from build123d import *

# Parameters (mm, degrees)
F1_DEPTH = 25.4


with BuildPart() as f1:
    # F0 (on Front) → F1 (new body)
    with BuildSketch(Plane.XZ):
        with BuildLine():
            Line((-180.280449281, -69.793186067), (-37.9985533655, -73.516196597))
            Line((-37.9985533655, -73.516196597), (-37.9985533655, -53.3922091126))
            ThreePointArc((-37.9985533655, -53.3922091126), (-36.3574166334, -49.6531424612), (-32.4943724898, -48.3299496779))
            Line((-32.4943724898, -48.3299496779), (32.4792108915, -48.1490081299))
            ThreePointArc((32.4792108915, -48.1490081299), (36.3518127667, -49.4657614096), (37.9985533655, -53.209974262))
            Line((37.9985533655, -53.209974262), (37.9985533655, -73.516196597))
            Line((37.9985533655, -73.516196597), (180.280449281, -69.793186067))
            Line((180.280449281, -69.793186067), (179.7684819711, -50.3384282921))
            ThreePointArc((179.7684819711, -50.3384282921), (181.2076799987, -46.6602509384), (184.8467238815, -45.124790347))
            Line((184.8467238815, -45.124790347), (224.0474202454, -45.124790347))
            ThreePointArc((224.0474202454, -45.124790347), (227.6395226938, -46.6126878986), (229.1274202454, -50.204790347))
            Line((229.1274202454, -50.204790347), (229.1274202454, -68.8998913716))
            Line((229.1274202454, -68.8998913716), (368.779072779, -65.2248478839))
            Line((368.779072779, -65.2248478839), (368.2445209989, -44.9118802426))
            ThreePointArc((368.2445209989, -44.9118802426), (369.6374073208, -41.2818793035), (373.1891249642, -39.7000003873))
            Line((373.1891249642, -39.7000003873), (413.8150602467, -38.6308968272))
            ThreePointArc((413.8150602467, -38.6308968272), (417.4450611859, -40.0237831491), (419.0269401021, -43.5755007925))
            Line((419.0269401021, -43.5755007925), (419.5614918821, -63.8884684338))
            Line((419.5614918821, -63.8884684338), (572.7053844218, -59.8583659985))
            Line((572.7053844218, -59.8583659985), (571.7030998342, -21.7715516712))
            ThreePointArc((571.7030998342, -21.7715516712), (573.0959861561, -18.141550732), (576.6477037995, -16.5596718159))
            Line((576.6477037995, -16.5596718159), (593.6560001815, -16.112085069))
            add(Edge.make_bspline(
                [(593.6560001815, -16.112085069), (596.1080901801, 20.5341002257), (601.6949471336, 104.0289944805), (592.471101525, 224.502637459), (587.295632267, 292.1)],
                knots=[0, 0, 0, 0, 0.4389033081, 1, 1, 1, 1], degree=3))
            Line((587.295632267, 292.1), (561.895632267, 292.1))
            ThreePointArc((561.895632267, 292.1), (555.545632267, 298.45), (561.895632267, 304.8))
            Line((561.895632267, 304.8), (561.895632267, 317.5))
            Line((561.895632267, 317.5), (479.345632267, 330.2))
            Line((479.345632267, 330.2), (479.345632267, 266.595095396))
            add(Edge.make_bspline(
                [(479.345632267, 266.595095396), (537.2284650803, 211.8650227785), (542.5910949707, 164.6739989519), (523.795632267, 101.6)],
                knots=[0, 0, 0, 0, 170.8776872642, 170.8776872642, 170.8776872642, 170.8776872642], degree=3))
            Line((523.795632267, 101.6), (479.345632267, 0))
            Line((479.345632267, 0), (0, 0))
            Line((0, 0), (-479.345632267, 0))
            Line((-479.345632267, 0), (-523.795632267, 101.6))
            add(Edge.make_bspline(
                [(-479.345632267, 266.595095396), (-537.2284650803, 211.8650227785), (-542.5910949707, 164.6739989519), (-523.795632267, 101.6)],
                knots=[0, 0, 0, 0, 170.8776872642, 170.8776872642, 170.8776872642, 170.8776872642], degree=3))
            Line((-479.345632267, 266.595095396), (-479.345632267, 330.2))
            Line((-479.345632267, 330.2), (-561.895632267, 317.5))
            Line((-561.895632267, 317.5), (-561.895632267, 304.8))
            ThreePointArc((-561.895632267, 304.8), (-555.545632267, 298.45), (-561.895632267, 292.1))
            Line((-561.895632267, 292.1), (-587.295632267, 292.1))
            add(Edge.make_bspline(
                [(-593.6560001815, -16.112085069), (-596.1080901801, 20.5341002257), (-601.6949471336, 104.0289944805), (-592.471101525, 224.502637459), (-587.295632267, 292.1)],
                knots=[0, 0, 0, 0, 0.4389033081, 1, 1, 1, 1], degree=3))
            Line((-593.6560001815, -16.112085069), (-576.6477037995, -16.5596718159))
            ThreePointArc((-576.6477037995, -16.5596718159), (-573.0959861561, -18.141550732), (-571.7030998342, -21.7715516712))
            Line((-571.7030998342, -21.7715516712), (-572.7053844218, -59.8583659985))
            Line((-572.7053844218, -59.8583659985), (-419.5614918821, -63.8884684338))
            Line((-419.5614918821, -63.8884684338), (-419.0269401021, -43.5755007925))
            ThreePointArc((-419.0269401021, -43.5755007925), (-417.4450611859, -40.0237831491), (-413.8150602467, -38.6308968272))
            Line((-413.8150602467, -38.6308968272), (-373.1891249642, -39.7000003873))
            ThreePointArc((-373.1891249642, -39.7000003873), (-369.6374073208, -41.2818793035), (-368.2445209989, -44.9118802426))
            Line((-368.2445209989, -44.9118802426), (-368.779072779, -65.2248478839))
            Line((-368.779072779, -65.2248478839), (-229.1274202454, -68.8998913716))
            Line((-229.1274202454, -68.8998913716), (-229.1274202454, -50.204790347))
            ThreePointArc((-229.1274202454, -50.204790347), (-227.6395226938, -46.6126878986), (-224.0474202454, -45.124790347))
            Line((-224.0474202454, -45.124790347), (-184.8467238815, -45.124790347))
            ThreePointArc((-184.8467238815, -45.124790347), (-181.2076799987, -46.6602509384), (-179.7684819711, -50.3384282921))
            Line((-179.7684819711, -50.3384282921), (-180.280449281, -69.793186067))
        make_face()
    extrude(amount=F1_DEPTH)


solid = f1.part
Verification items for the finished model (mm, model axes). A direction names the side the tool comes from. Give positions to 0.01 mm unless a question says otherwise; leave off trailing zeros. Write each loop counter-clockwise with the first axis right and the second up, starting at its lowest first coordinate (ties: lowest second). Pieces come first, ordered by that corner, then holes.
(1) Access from +Z, -Z, +X, -X, +Y, -Y to the whole of each face (thin tool, end or side, straight path). Record for faces 4 (the face through (-479.346, -13, 298)), 5 (the face through (575, -13, 292.1)), 6 (the face through (204, -13, -45.125)).
(2) Mould release check, pull along Z, two halves, no side actions. Record for faces 1 (the face through (479.346, -13, 299)), 2 (the face through (501.88, -12.52, 51.51)), 3 (the face through (-574, -13, 292.1)): +Z half, -Z half, draft (parallel to the pull), parting line (faces both ways), or undercut.
(3) Cross-section at A-A (x = 160). Enter the section's corners in (y, z).
(4) Material ranges on line 1 (X direction, y = -24, z = -52.5); line 2 (X direction, y = -23.75, z = 230.5); line 3 (Z direction, x = -511, y = -18.5), recorded low to high.
(5) Cross-section at B-B (x = -161). Enter the section's corners in (y, z).
(6) Gauge pin test, flat ends, axial feed: pin 1 (9.5 mm diameter, centred on y = -11, z = -62.5, fed in from -X); pin 2 (1 mm diameter, centred on x = 264, y = -15, fed in from -Z); pin 3 (12.5 mm diameter, centred on y = -15, z = 312, fed in from -X). Record the tip position at first contact, or that the pin passes through.
Worked out:
1. face 4: +Z, +Y, -Y
1. face 5: +Z, +X, +Y, -Y
1. face 6: -Z, +Y, -Y
2. face 1: draft
2. face 2: undercut
2. face 3: +Z half
3. outline: (-25.4, -70.32) - (0, -70.32) - (0, 0) - (-25.4, 0) - close
4. line 1: x = -572.51 to -419.26, -368.44 to -229.13, -179.83 to -37.92, 37.95 to 179.83, 229.13 to 368.44, 419.26 to 572.51
4. line 2: x = -591.9 to -510.78, 510.78 to 591.9
4. line 3: z = -61.48 to 72.35, 230.18 to 325.33
5. outline: (-25.4, -70.3) - (0, -70.3) - (0, 0) - (-25.4, 0) - close
6. pin 1: stops at x = -572.71
6. pin 2: stops at z = -68
6. pin 3: stops at x = -561.9
